from build123d import *

# Parameters (mm, degrees)
SKETCH_R        = 55
PAD_DEPTH       = 40
POCKET_DEPTH    = 22
POCKET001_DEPTH = 16
SKETCH004_R     = 68.724133
SKETCH004_R_2   = 60.683335
POCKET002_DEPTH = 0.5


with BuildPart() as part:
    # Sketch → Pad (new body)
    with BuildSketch(Plane.XZ):
        with BuildLine():
            Line((-120, 75), (0, 75))
            ThreePointArc((-74.66808, -7.048245), (55.468993, -50.479608), (0, 75))
            ThreePointArc((-74.66808, -7.048245), (-83.30852, 13.959176), (-102.203647, 26.566441))
            ThreePointArc((-120, 50.506104), (-115.063539, 35.591198), (-102.203647, 26.566441))
            Line((-120, 75), (-120, 50.506104))
        make_face()
        Circle(SKETCH_R, mode=Mode.SUBTRACT)
    extrude(amount=PAD_DEPTH)

    # Sketch001 (on Face7 of Pad) → Pocket (cut)
    with BuildSketch(Plane(origin=(0, 0, 0), x_dir=(1, 0, 0), z_dir=(0, 1, 0))):
        with BuildLine():
            Line((52.081201, -18.140076), (85.552432, -51.611306))
            ThreePointArc((85.552432, -51.611306), (26.786197, 96.257182), (-99.914691, 0))
            Line((-211.758942, -108.831918), (-99.914691, 0))
            Line((-54.008053, -108.831918), (-211.758942, -108.831918))
            Line((-37.907945, -48.745498), (-54.008053, -108.831918))
            Line((18.140076, -52.081201), (-37.907945, -48.745498))
            Line((52.081201, -18.140076), (18.140076, -52.081201))
        make_face()
    extrude(amount=-POCKET_DEPTH, mode=Mode.SUBTRACT)

    # Sketch003 (on Face2 of Pocket) → Pocket001 (cut)
    with BuildSketch(Plane(origin=(0, -22, 0), x_dir=(1, 0, 0), z_dir=(0, 1, 0))):
        with BuildLine():
            ThreePointArc((0, -70), (66.404243, -22.146705), (42.018147, 55.986385))
            Line((42.018147, 55.986385), (62.226624, 86.16832))
            Line((62.226624, 86.16832), (-170.809082, 86.16832))
            Line((-170.809082, 86.16832), (-170.809082, -70))
            Line((-170.809082, -70), (0, -70))
        make_face()
    extrude(amount=-POCKET001_DEPTH, mode=Mode.SUBTRACT)

    # Sketch004 → Pocket002 (cut)
    with BuildSketch(Plane(origin=(0, -38, 0), x_dir=(-1, 0, 0), z_dir=(0, 1, 0))):
        Circle(SKETCH004_R)
        Circle(SKETCH004_R_2, mode=Mode.SUBTRACT)
    extrude(amount=-POCKET002_DEPTH, mode=Mode.SUBTRACT)


solid = part.part
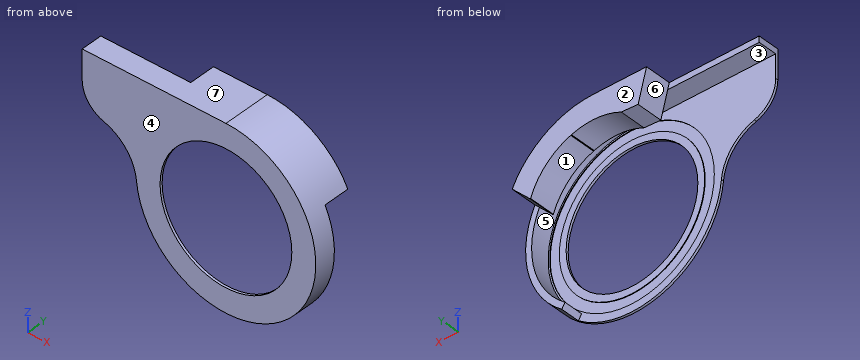
Build history of the part. All positions in model axes, mm. Face numbers are marked on the shaded views. A direction names the side the tool comes from. Coordinates: 2 decimals unless noted, no trailing zeros. Order: outer loops, then holes, each group sorted by start corner. A loop starts at its lowest first (then second) coordinate and runs counter-clockwise, first axis right, second up. Notation, with made-up numbers: (7.25, -10.75) -> (46.25, -10.75) arc R20 cw to (46.25, 17.25) -> close; hole circle Ø11 at (80, 33). An arc over 180 degrees is marked (long way). One line per item, written item: value.
(1) Mould opens along Y. For the marked faces 1, 2, 3 and 4 say: pulls with the +Y half, pulls with the -Y half, needs draft (parallel to the pull), parting line crosses it, or undercut.
Checked values:
face 1: needs draft
face 2: pulls with the +Y half
face 3: undercut
face 4: pulls with the -Y half
(2) Drop flat-ended pins along their axis: pin 1 Ø13 at (x, y) = (-72, -29.5) entering from -Z; pin 2 Ø16.5 at (x, z) = (52.5, -29) entering from +Y; pin 3 Ø6 at (x, y) = (28, -12) entering from -Z; pin 4 Ø1.5 at (y, z) = (-21, -48.5) entering from +X. Give the stop position or say it passes through.
Checked values:
pin 1: z = 70
pin 2: y = -38
pin 3: z = 45.43
pin 4: through
(3) Slice it at C-C, the plane x = 13. List the corners of the cut face in (y, z), plus the area to 3 significant figures.
Checked values:
outline: (-40, -73.86) -> (-38, -73.86) -> (-38, -67.48) -> (-38.5, -67.48) -> (-38.5, -59.27) -> (-38, -59.27) -> (-38, -53.44) -> (-40, -53.44) -> close; (-40, 53.44) -> (-38, 53.44) -> (-38, 59.27) -> (-38.5, 59.27) -> (-38.5, 67.48) -> (-38, 67.48) -> (-38, 68.78) -> (-22, 68.78) -> (-22, 53.44) -> (0, 53.44) -> (0, 73.86) -> (-40, 73.86) -> close
area: 604 mm2
(4) Slice it at B-B, the plane y = -16.5. List the corners of the cut face in (x, z).
Checked values:
outline: (-44.94, 75) -> (-37.91, 48.75) -> (-23.8, 49.59) arc R55 cw to (17.75, 52.06) -> (18.14, 52.08) -> (18.39, 51.84) arc R55 cw to (51.84, 18.39) -> (52.08, 18.14) -> (67.21, 33.27) arc R75 ccw to (0, 75) -> close
(5) Tool access for the marked faces 5, 6 and 7: list every direction of +Z, -Z, +X, -X, +Y, -Y with a clear straight run to the whole face (end or side of a thin tool).
Checked values:
face 5: -X
face 6: -Z, -X, +Y
face 7: +Z, +X, -X, +Y, -Y
(6) Probe line 1 (Y direction, x = -81.5, z = 47.5); line 2 (X direction, y = -39, z = 0); line 3 (Y direction, x = -61.5, z = 8). List the from-to ranges inside material, lowest first. Write a range as [from, to].
Checked values:
line 1: [-40, -38]
line 2: [-76, -55], [55, 75]
line 3: [-40, -38.5]
(7) Slice it at D-D, the plane z = 0. List the corners of the cut face in (x, y).
Checked values:
outline: (-76, -40) -> (-55, -40) -> (-55, -38) -> (-60.68, -38) -> (-60.68, -38.5) -> (-68.72, -38.5) -> (-68.72, -38) -> (-76, -38) -> close; (55, -40) -> (75, -40) -> (75, -22) -> (70, -22) -> (70, -38) -> (68.72, -38) -> (68.72, -38.5) -> (60.68, -38.5) -> (60.68, -38) -> (55, -38) -> close
(8) Slice it at A-A, the plane z = -42.5. List the corners of the cut face in (x, y), plus the area to 3 significant figures.
Checked values:
outline: (-61.8, -40) -> (-34.91, -40) -> (-34.91, -38) -> (-43.32, -38) -> (-43.32, -38.5) -> (-54.01, -38.5) -> (-54.01, -38) -> (-61.8, -38) -> close; (34.91, -40) -> (61.8, -40) -> (61.8, -22) -> (55.62, -22) -> (55.62, -38) -> (54.01, -38) -> (54.01, -38.5) -> (43.32, -38.5) -> (43.32, -38) -> (34.91, -38) -> close
area: 196 mm2
